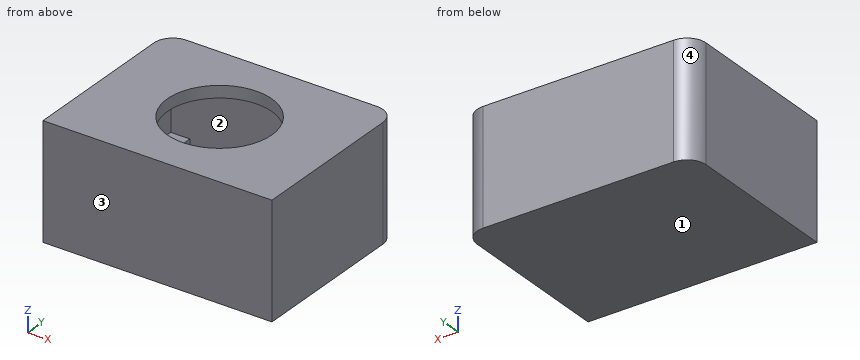
Autodesk Inventor part; units mm, degrees
ref_plane "YZ Plane" through (0, 0, 0) normal (1, 0, 0) x (0, 1, 0)
ref_plane "XZ Plane" through (0, 0, 0) normal (0, 1, 0) x (-1, 0, 0)
ref_plane "XY Plane" through (0, 0, 0) normal (0, 0, 1) x (1, 0, 0)
sketch "Sketch1" plane through (0, 0, 0) normal (0, 1, 0) x (-1, 0, 0)
  line L0 (152.4, 76.2) -> (-152.4, 76.2)
  line L1 (-152.4, 76.2) -> (-152.4, -76.2)
  line L2 (-152.4, -76.2) -> (152.4, -76.2)
  line L3 (152.4, -76.2) -> (152.4, 76.2)
  point P0 (0, 0)
  point P1 (152.4, 0)
  point P2 (0, -76.2)
  dimension "d0" = 152.4
  dimension "d1" = 304.8
extrude "Extrusion1" add sketch "Sketch1" along normal blind 15.875
sketch "Sketch4" plane through (0, 15.875, 0) normal (0, 1, 0) x (1, 0, 0)
  line L0 (-152.4, -76.2) -> (152.4, -76.2)
  line L1 (152.4, -76.2) -> (152.4, 76.2)
  line L2 (152.4, 76.2) -> (-152.4, 76.2)
  line L3 (-152.4, 76.2) -> (-152.4, -76.2)
  line L4 (-152.4, -76.2) -> (152.4, -76.2)
  line L5 (-152.4, -76.2) -> (136.525, -76.2)
  line L6 (136.525, -76.2) -> (136.525, -60.325)
  line L7 (136.525, -60.325) -> (-152.4, -60.325)
  line L8 (-152.4, -60.325) -> (-152.4, -76.2)
  point P0 (0, 0)
  dimension "d4" = 15.875
  dimension "d5" = 15.875
extrude "Extrusion2" add sketch "Sketch4" along normal blind 203.2 contours L3 L7 L6 L0
sketch "Sketch5" plane through (0, 15.875, 0) normal (0, 1, 0) x (1, 0, 0)
  line L0 (136.525, -60.325) -> (136.525, -76.2)
  line L1 (136.525, -76.2) -> (152.4, -76.2)
  line L2 (152.4, -76.2) -> (152.4, 76.2)
  line L3 (152.4, 76.2) -> (-152.4, 76.2)
  line L4 (-152.4, 76.2) -> (-152.4, -60.325)
  line L5 (-152.4, -60.325) -> (136.525, -60.325)
  line L6 (-152.4, -76.2) -> (152.4, -76.2)
  line L7 (152.4, -76.2) -> (136.525, -76.2)
  line L8 (136.525, -76.2) -> (136.525, 60.325)
  line L9 (136.525, 60.325) -> (152.4, 60.325)
  line L10 (152.4, 60.325) -> (152.4, -76.2)
  line L11 (136.525, -76.2) -> (136.525, -60.325)
  point P0 (0, 0)
  dimension "d8" = 15.875
extrude "Extrusion3" add sketch "Sketch5" along normal blind 203.2 contours L8 L9 L2 L1 L0
sketch "Sketch6" plane through (0, 15.875, 0) normal (0, 1, 0) x (1, 0, 0)
  line L0 (136.525, 60.325) -> (152.4, 60.325)
  line L1 (152.4, 60.325) -> (152.4, 76.2)
  line L2 (152.4, 76.2) -> (-152.4, 76.2)
  line L3 (-152.4, 76.2) -> (-152.4, -60.325)
  line L4 (-152.4, -60.325) -> (136.525, -60.325)
  line L5 (136.525, -60.325) -> (136.525, 60.325)
  line L6 (152.4, 76.2) -> (-136.525, 76.2)
  line L7 (-136.525, 76.2) -> (-136.525, 60.325)
  line L8 (-136.525, 60.325) -> (152.4, 60.325)
  line L9 (152.4, 60.325) -> (152.4, 76.2)
  line L10 (152.4, 60.325) -> (136.525, 60.325)
  point P0 (0, 0)
  dimension "d11" = 15.875
extrude "Extrusion4" add sketch "Sketch6" along normal blind 203.2 contours L8 L7 L2 L1 L0
sketch "Sketch7" plane through (0, 15.875, 0) normal (0, 1, 0) x (1, 0, 0)
  line L0 (-136.525, 60.325) -> (-136.525, 76.2)
  line L1 (-136.525, 76.2) -> (-152.4, 76.2)
  line L2 (-152.4, 76.2) -> (-152.4, -60.325)
  line L3 (-152.4, -60.325) -> (136.525, -60.325)
  line L4 (136.525, -60.325) -> (136.525, 60.325)
  line L5 (136.525, 60.325) -> (-136.525, 60.325)
  line L6 (-152.4, -60.325) -> (136.525, -60.325)
  line L7 (-152.4, 76.2) -> (-136.525, 76.2)
  line L8 (-136.525, 76.2) -> (-136.525, -60.325)
  line L9 (-136.525, -60.325) -> (-152.4, -60.325)
  line L10 (-152.4, -60.325) -> (-152.4, 76.2)
  line L11 (-136.525, 76.2) -> (-136.525, 60.325)
  point P0 (0, 0)
extrude "Extrusion5" add sketch "Sketch7" along normal blind 203.2 contours L8 L3 L2 L1 L0
sketch "Sketch8" plane through (0, 219.075, 0) normal (0, 1, 0) x (1, 0, 0)
  line L0 (136.525, -60.325) -> (-136.525, -60.325)
  line L1 (-152.4, 76.2) -> (-152.4, -76.2)
  line L2 (152.4, -76.2) -> (152.4, 76.2)
  line L3 (-152.4, 76.2) -> (152.4, 76.2)
  line L4 (152.4, 76.2) -> (152.4, -76.2)
  line L5 (152.4, -76.2) -> (-152.4, -76.2)
  line L6 (-152.4, -76.2) -> (-152.4, 76.2)
  line L7 (-152.4, -76.2) -> (152.4, -76.2)
  line L8 (136.525, 60.325) -> (136.525, -60.325)
  line L9 (152.4, -76.2) -> (152.4, 76.2)
  line L10 (-136.525, 60.325) -> (136.525, 60.325)
  line L11 (-136.525, -60.325) -> (-136.525, 60.325)
  line L12 (152.4, 76.2) -> (-152.4, 76.2)
  point P0 (0, 0)
extrude "Extrusion6" add sketch "Sketch8" along normal blind 15.875 contours L0 L11 L10 L8 | L3 L2 L5 L1
sketch "Sketch9" plane through (-152.4, 0, 76.2) normal (0, 0, 1) x (1, 0, 0)
  circle A0 centre (152.4, 117.475) radius 69.5
  line L0 (0, 0) -> (304.8, 0)
  line L1 (304.8, 0) -> (304.8, 234.95)
  line L2 (0, 0) -> (0, 234.95)
  line L3 (0, 234.95) -> (304.8, 234.95)
  line L4 (0, 234.95) -> (304.8, 234.95)
  point P0 (152.4, 0)
  point P1 (304.8, 117.475)
  point P2 (152.4, 234.95)
  point P3 (234.95, 190.5)
  point P4 (152.4, 234.95)
  dimension "d18" = 139
extrude "Extrusion7" cut sketch "Sketch9" against normal up to next contours A0
sketch "Sketch10" plane through (0, 15.875, 0) normal (0, 1, 0) x (1, 0, 0)
  line L0 (-136.525, 60.325) -> (-136.525, -60.325)
  line L1 (-136.525, -60.325) -> (136.525, -60.325)
  line L2 (136.525, -60.325) -> (136.525, 60.325)
  line L3 (136.525, 60.325) -> (-136.525, 60.325)
  line L4 (-136.525, 60.325) -> (-111.125, 60.325)
  line L5 (-111.125, 60.325) -> (-111.125, 34.925)
  line L6 (-111.125, 34.925) -> (-136.525, 34.925)
  line L7 (-136.525, 34.925) -> (-136.525, 60.325)
  line L8 (136.525, 60.325) -> (111.125, 60.325)
  line L9 (111.125, 60.325) -> (111.125, 34.925)
  line L10 (111.125, 34.925) -> (136.525, 34.925)
  line L11 (136.525, 34.925) -> (136.525, 60.325)
  line L12 (-136.525, -60.325) -> (-111.125, -60.325)
  line L13 (-111.125, -60.325) -> (-111.125, -34.925)
  line L14 (-111.125, -34.925) -> (-136.525, -34.925)
  line L15 (-136.525, -34.925) -> (-136.525, -60.325)
  line L16 (136.525, -60.325) -> (111.125, -60.325)
  line L17 (111.125, -60.325) -> (111.125, -34.925)
  line L18 (111.125, -34.925) -> (136.525, -34.925)
  line L19 (136.525, -34.925) -> (136.525, -60.325)
  point P0 (0, 0)
  dimension "d21" = 25.4
  dimension "d22" = 25.4
  dimension "d23" = 25.4
  dimension "d24" = 25.4
  dimension "d25" = 25.4
  dimension "d26" = 25.4
extrude "Extrusion8" add sketch "Sketch10" along normal up to surface (203.2 mm away) contours L3 L5 L6 L0 | L14 L13 L1 L0 | L3 L2 L10 L9 | L17 L18 L2 L1
fillet "Fillet1" radius 25.4 2 edges at (152.4, 234.95, 0) (-152.4, 234.95, 0)
equation "\"d5\" = d4"
properties part number "speakerBox" material "Wood (Birch)"
For this review, take the finished solid that the model builds, in its own axes (mm). Face numbers are marked on the shaded views. Give positions to 0.01 mm unless a question says otherwise; leave off trailing zeros. Order: outer loops, then holes, each group sorted by start corner. A loop starts at its lowest first (then second) coordinate and runs counter-clockwise, first axis right, second up.
1) Take a section at D-D (y = 132.5). Give the boundary of the cut face in (x, z) (3 decimals), then the cut area to 3 significant figures.
2) Take a section at C-C (x = 0). Give the boundary of the cut face in (y, z) (3 decimals), then the cut area to 3 significant figures.
3) The part is to be moulded in two halves that separate along Y. For the marked faces 1, 2, 3 and 4, say which applies: released by +Y, released by -Y, zero draft, split by the parting line, or undercut.
4) Wall thickness on line 1 (Y direction, x = 56, z = 59.5) (3 decimals); line 2 (Z direction, x = -38.5, y = 178) (3 decimals); line 3 (Z direction, x = -115.5, y = 196) (3 decimals): over which ranges is each line inside the solid? List them lowest first.
5) Take a section at B-B (x = -103.5). Give the boundary of the cut face in (y, z) (3 decimals), then the cut area to 3 significant figures.
6) Take a section at A-A (z = -53.5). Give the boundary of the cut face in (x, y) (3 decimals).
Derived:
1. outline: (-152.4, -76.2) - (152.4, -76.2) - (152.4, 76.2) - (67.856, 76.2) - (67.856, 60.325) - (111.125, 60.325) - (111.125, 34.925) - (136.525, 34.925) - (136.525, -34.925) - (111.125, -34.925) - (111.125, -60.325) - (-111.125, -60.325) - (-111.125, -34.925) - (-136.525, -34.925) - (-136.525, 34.925) - (-111.125, 34.925) - (-111.125, 60.325) - (-67.856, 60.325) - (-67.856, 76.2) - (-152.4, 76.2) - close
1. area: 13,900 mm2
2. outline: (0, -76.2) - (234.95, -76.2) - (234.95, 76.2) - (186.975, 76.2) - (186.975, 60.325) - (219.075, 60.325) - (219.075, -60.325) - (15.875, -60.325) - (15.875, 60.325) - (47.975, 60.325) - (47.975, 76.2) - (0, 76.2) - close
2. area: 9,080 mm2
3. face 1: zero draft
3. face 2: undercut
3. face 3: released by -Y
3. face 4: released by +Y
4. line 1: y = 0 to 15.875, 219.075 to 234.95
4. line 2: z = -76.2 to -60.325, 60.325 to 76.2
4. line 3: z = -76.2 to -34.925, 34.925 to 76.2
5. outline: (0, -76.2) - (234.95, -76.2) - (234.95, 76.2) - (0, 76.2) - close; hole (15.875, -60.325) - (219.075, -60.325) - (219.075, 60.325) - (15.875, 60.325) - close
5. area: 11,300 mm2
6. outline: (-152.4, 0) - (152.4, 0) - (152.4, 209.55) arc R25.4 ccw to (127, 234.95) - (-127, 234.95) arc R25.4 ccw to (-152.4, 209.55) - close; hole (-111.125, 15.875) - (111.125, 15.875) - (111.125, 219.075) - (-111.125, 219.075) - close
